from build123d import *

# Parameters (mm, degrees)
SKETCH1_R                = 13.442813203
BOSS_EXTRUDE1_DEPTH      = 2
SKETCH2_W                = 6.5
SKETCH2_H                = 18
SKETCH2_W_2              = 3
SKETCH2_H_2              = 14.5
BOSS_EXTRUDE3_DEPTH      = 2
FILLET1_R                = 1.5
CIRPATTERN1_COUNT        = 4
FILLET1_OF_CIRPATTERN1_R = 1.5
SKETCH3_R                = 6
SKETCH3_R_2              = 4.5
BOSS_EXTRUDE4_DEPTH      = 18
FILLET2_R                = 4


with BuildPart() as part:
    # Sketch1 → Boss-Extrude1 (new body)
    with BuildSketch(Plane(origin=(0, 0, 0), x_dir=(1, 0, 0), z_dir=(0, 1, 0))):
        with Locations(Location((0, 0, 0), (0, 0, 270))):
            Circle(SKETCH1_R)
    extrude(amount=BOSS_EXTRUDE1_DEPTH)

    # Sketch2 → Boss-Extrude3 (add)
    with BuildSketch(Plane(origin=(0, 2, 0), x_dir=(1, 0, 0), z_dir=(0, 1, 0))):
        with Locations((0, 13.442813203)):
            Rectangle(SKETCH2_W, SKETCH2_H)
        with Locations((0, 13.442813203)):
            Rectangle(SKETCH2_W_2, SKETCH2_H_2, mode=Mode.SUBTRACT)
    boss_extrude3 = extrude(amount=-BOSS_EXTRUDE3_DEPTH)

    # Fillet1
    fillet1_edges = [part.edges().sort_by_distance(p)[0] for p in [
        (3.25, 1, -13.044030313),
        (3.25, 1, -22.442813203),
        (-3.25, 1, -22.442813203),
        (-3.25, 1, -13.044030313),
        (-1.5, 1, -13.35886323),
        (1.5, 1, -13.35886323),
        (1.5, 1, -20.692813203),
        (-1.5, 1, -20.692813203),
    ]]
    fillet(fillet1_edges, radius=FILLET1_R - 0.0001)  # a hair under: the kernel refuses the full size

    # CirPattern1: Boss-Extrude3 ×4 about axis
    cirpattern1_axis = Axis((0, 0, 0), (0, 1, 0))
    for i in range(1, CIRPATTERN1_COUNT):
        add(boss_extrude3.rotate(cirpattern1_axis, i * 360 / CIRPATTERN1_COUNT))

    # Fillet1 of CirPattern1
    fillet1_of_cirpattern1_edges = [part.edges().sort_by_distance(p)[0] for p in [
        (-13.044030313, 1, -3.25),
        (-22.442813203, 1, -3.25),
        (-22.442813203, 1, 3.25),
        (-13.044030313, 1, 3.25),
        (-13.35886323, 1, 1.5),
        (-13.35886323, 1, -1.5),
        (-20.692813203, 1, -1.5),
        (-20.692813203, 1, 1.5),
        (-3.25, 1, 13.044030313),
        (-3.25, 1, 22.442813203),
        (3.25, 1, 22.442813203),
        (3.25, 1, 13.044030313),
        (1.5, 1, 13.35886323),
        (-1.5, 1, 13.35886323),
        (-1.5, 1, 20.692813203),
        (1.5, 1, 20.692813203),
        (13.044030313, 1, 3.25),
        (22.442813203, 1, 3.25),
        (22.442813203, 1, -3.25),
        (13.044030313, 1, -3.25),
        (13.35886323, 1, -1.5),
        (13.35886323, 1, 1.5),
        (20.692813203, 1, 1.5),
        (20.692813203, 1, -1.5),
    ]]
    fillet(fillet1_of_cirpattern1_edges, radius=FILLET1_OF_CIRPATTERN1_R - 0.0001)  # a hair under: the kernel refuses the full size

    # Sketch3 → Boss-Extrude4 (add)
    with BuildSketch(Plane(origin=(0, 2, 0), x_dir=(1, 0, 0), z_dir=(0, 1, 0))):
        with Locations(Location((0, 0, 0), (0, 0, 270))):
            Circle(SKETCH3_R)
        with Locations(Location((0, 0, 0), (0, 0, 270))):
            Circle(SKETCH3_R_2, mode=Mode.SUBTRACT)
    extrude(amount=BOSS_EXTRUDE4_DEPTH)

    # Fillet2
    fillet2_edges = [part.edges().sort_by_distance(p)[0] for p in [
        (0, 2, -6),
    ]]
    fillet(fillet2_edges, radius=FILLET2_R)


solid = part.part
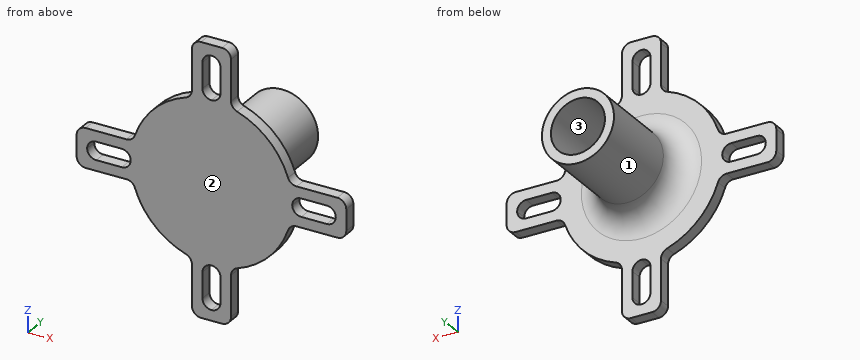
Read the model definition and answer for the solid it produces. Units are mm, in the model's axes. Face numbers are marked on the shaded views. Give positions to 0.01 mm unless a question says otherwise; leave off trailing zeros. Loops run counter-clockwise (first coordinate to the right, second up) from the corner with the lowest first, then second, coordinate; pieces in that order, holes last. Notation, with made-up numbers: (-16.75, 88.25) - (22.25, 88.25) arc R16 ccw to (22.25, 104.25) - close; hole circle Ø10 at (82, 59). An arc over 180 degrees is marked (long way). Answer as CSV lines item,"result". Start each with the question number.
1) Each of these flat-tipped pins is pushed along its axis until it touches: pin 1 Ø8 at (x, y) = (10.5, 10.5) entering from -Z; pin 2 Ø1 at (y, z) = (14, 2.5) entering from +X; pin 3 Ø1 at (y, z) = (0.5, 16.5) entering from +X; pin 4 Ø1 at (x, y) = (17.5, 1.5) entering from -Z. Where does it stop, or does it pass through?
2) Find section B-B (y = 7). Write down the section's boundary in (x, z), then the cut area to 3 significant figures.
3) Straight lines are drawn through the part: L1, parallel to X at y = 15, z = 0; L2, parallel to X at y = 17.25, z = 1. For each, find the intervals that lie inside material, in ascending order. Write a range as from..to.
4) Find section A-A (x = 15.5). Write down the section's boundary in (y, z).
5) Determine the mould class of the marked faces 1, 2 and 3 for opening direction X: released by +X, released by -X, zero draft, split by the parting line, or undercut.
6) Find section C-C (y = 2.75). Write down the section's boundary in (x, z).
Findings below:
1,pin 1,"through"
1,pin 2,"x = 5.66"
1,pin 3,"x = 3.25"
1,pin 4,"z = -3.25"
2,outline,"circle Ø12 at (0, 0); hole circle Ø9 at (0, 0)"
2,area,"49.5 mm^2"
3,L1,"-6..-4.5, 4.5..6"
3,L2,"-5.92..-4.39, 4.39..5.92"
4,outline,"(0, -3.25) - (2, -3.25) - (2, -1.5) - (0, -1.5) - close; (0, 1.5) - (2, 1.5) - (2, 3.25) - (0, 3.25) - close"
5,face 1,"split by the parting line"
5,face 2,"zero draft"
5,face 3,"undercut"
6,outline,"circle Ø15.34 at (0, 0); hole circle Ø9 at (0, 0)"
